from build123d import *

# Parameters (mm, degrees)
BOSS_EXTRU_1_DEPTH      = 6
BOSS_EXTRU_2_DEPTH      = 12
ESQUISSE14_W            = 21
ESQUISSE14_H            = 6
ENL_V_MAT_EXTRU_2_DEPTH = 21
D_GAGEMENT_M81_D        = 9
TROU_TARAUD_M82_D       = 6.8
CONG_1_R                = 2


with BuildPart() as part:
    # Esquisse1 → Boss.-Extru.1 (new body)
    with BuildSketch(Plane(origin=(0, 0, 0), x_dir=(1, 0, 0), z_dir=(0, 1, 0))):
        with BuildLine():
            Line((0, 0), (0, 30))
            ThreePointArc((0, 30), (10, 40), (20, 30))
            Line((20, 30), (20, 0))
            ThreePointArc((20, 0), (10, -10), (0, 0))
        make_face()
    extrude(amount=BOSS_EXTRU_1_DEPTH)

    # Esquisse12 → Boss.-Extru.2 (add)
    with BuildSketch(Plane.XZ):
        with BuildLine():
            Line((0, -30), (20, -30))
            Line((20, -30), (20, 0))
            ThreePointArc((20, 0), (10, 10), (0, 0))
            Line((0, 0), (0, -30))
        make_face()
    extrude(amount=BOSS_EXTRU_2_DEPTH)

    # Esquisse14 → Enlèv. mat.-Extru.2 (cut, through all)
    with BuildSketch(Plane(origin=(20, 0, 0), x_dir=(0, 0, -1), z_dir=(1, 0, 0))):
        with Locations((0.5, 3)):
            Rectangle(ESQUISSE14_W, ESQUISSE14_H)
        Polygon((30, 0), (19, 0), (19, -6), (-10, -6), (-10, -12), (30, -12), align=None)
    extrude(amount=-ENL_V_MAT_EXTRU_2_DEPTH, mode=Mode.SUBTRACT)

    # Dégagement M81 (through all)
    with Locations(Plane(origin=(0, 6, 0), x_dir=(1, 0, 0), z_dir=(0, 1, 0))):
        with Locations((10, 30)):
            Hole(D_GAGEMENT_M81_D / 2)

    # Trou taraudé M82 (through all)
    with Locations(Plane(origin=(0, 0, 0), x_dir=(1, 0, 0), z_dir=(0, 1, 0))):
        with Locations((10, 0)):
            Hole(TROU_TARAUD_M82_D / 2)

    # Congé1
    cong_1_edges = [part.edges().sort_by_distance(p)[0] for p in [
        (10, -6, -19),
        (10, 6, -11),
    ]]
    fillet(cong_1_edges, radius=CONG_1_R)


solid = part.part
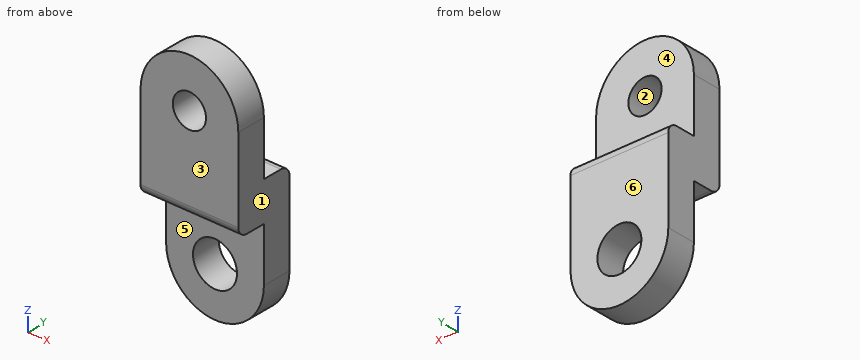
The listing builds one solid part. Answer for the finished solid, in the listing's coordinates (mm). Face numbers are marked on the shaded views. A direction names the side the tool comes from. Give positions to 0.01 mm unless a question says otherwise; leave off trailing zeros. Loops run counter-clockwise (first coordinate to the right, second up) from the corner with the lowest first, then second, coordinate; pieces in that order, holes last.
Item 1: Find the intervals of material crossed by line 1 along Z through (x, y) = (10, -3.6); line 2 along Z through (x, y) = (10, 2.6); line 3 along Y through (x, z) = (19.25, -5), in increasing order.
Derived:
line 1: z = -19 to -3.4, 3.4 to 10
line 2: z = -40 to -34.5, -25.5 to -11
line 3: y = -6 to 0
Item 2: A cutting plane is placed at A-A (x = 10). Give the vertices of the cut face in (y, z).
Derived:
outline: (-6, -17) arc R2 ccw to (-4, -19) - (0, -19) - (0, -25.5) - (6, -25.5) - (6, -13) arc R2 ccw to (4, -11) - (0, -11) - (0, -3.4) - (-6, -3.4) - close; (-6, 3.4) - (0, 3.4) - (0, 10) - (-6, 10) - close; (0, -40) - (6, -40) - (6, -34.5) - (0, -34.5) - close
Item 3: A tool of negligible diameter and unlimited length cuts with its end or side. For the marked faces 4, 5 and 6, from which of +Z, -Z, +X, -X, +Y, -Y can it reach the whole face along a straight path? Write none if from no direction.
Derived:
face 4: +Z, +X, -X, +Y
face 5: -Z, +X, -X, -Y
face 6: +Z, -Z, +X, -X, +Y
Item 4: Each of these flat-tipped pins is pushed along its axis until it touches: pin 1 Ø4.5 at (x, y) = (6, -2.5) entering from -Z; pin 2 Ø6 at (x, z) = (13, -0.5) entering from +Y; pin 3 Ø1.5 at (x, y) = (13.5, 0.5) entering from -Z; pin 4 Ø12 at (x, z) = (10, -29) entering from +Y. Where does it stop, or does it pass through?
Derived:
pin 1: stops at z = -19
pin 2: stops at y = 0
pin 3: stops at z = -39.61
pin 4: stops at y = 6
Item 5: Determine the mould class of the marked faces 1, 2 and 3 for opening direction X: +X half, -X half, draft (parallel to the pull), parting line (faces both ways), or undercut.
Derived:
face 1: +X half
face 2: undercut
face 3: draft
Item 6: A cutting plane is placed at B-B (z = -33). Give the vertices of the cut face in (x, y).
Derived:
outline: (0.46, 0) - (6.65, 0) - (6.65, 6) - (0.46, 6) - close; (13.35, 0) - (19.54, 0) - (19.54, 6) - (13.35, 6) - close
Item 7: A cutting plane is placed at C-C (y = 3). Give the vertices of the cut face in (x, z).
Derived:
outline: (0, -30) arc R10 ccw to (20, -30) - (20, -11) - (0, -11) - close; hole circle Ø9 at (10, -30)
Item 8: A cutting plane is placed at D-D (x = 2). Give the vertices of the cut face in (y, z).
Derived:
outline: (-6, -17) arc R2 ccw to (-4, -19) - (0, -19) - (0, -36) - (6, -36) - (6, -13) arc R2 ccw to (4, -11) - (0, -11) - (0, 6) - (-6, 6) - close
